```python
from build123d import *

# Parameters (mm, degrees)
SKETCH2_W           = 68.2625
SKETCH2_H           = 52.3875
BOSS_EXTRUDE1_DEPTH = 1.5875
SKETCH3_W           = 38.1
SKETCH3_H           = 3.175
SKETCH3_W_2         = 47.625
SKETCH3_W_3         = 4.7625
SKETCH3_H_2         = 7.9375
SKETCH3_W_4         = 7.9375
SKETCH3_H_3         = 4.7625
BOSS_EXTRUDE2_DEPTH = 7.9375
SKETCH5_W           = 34.925
SKETCH5_H           = 4.7625
BOSS_EXTRUDE3_DEPTH = 7.14375
FILLET1_R           = 1.27
SKETCH6_R           = 2.737420774
BOSS_EXTRUDE4_DEPTH = 6.35
SKETCH7_W           = 15.875
SKETCH7_H           = 12.7
BOSS_EXTRUDE5_DEPTH = 11.1125
SKETCH8_W           = 14.2875
SKETCH8_H           = 9.525
BOSS_EXTRUDE6_DEPTH = 11.1125
SKETCH9_R           = 1.5875
CUT_EXTRUDE1_DEPTH  = 1.5875


with BuildPart() as part:
    # Sketch2 → Boss-Extrude1 (new body)
    with BuildSketch(Plane(origin=(0, 0, 0), x_dir=(1, 0, 0), z_dir=(0, 1, 0))):
        with Locations((34.13125, 26.19375)):
            Rectangle(SKETCH2_W, SKETCH2_H)
    extrude(amount=BOSS_EXTRUDE1_DEPTH)

    # Sketch3 → Boss-Extrude2 (add)
    with BuildSketch(Plane(origin=(0, 1.5875, 0), x_dir=(1, 0, 0), z_dir=(0, 1, 0))):
        with Locations((22.225, 49.2125)):
            Rectangle(SKETCH3_W, SKETCH3_H)
        with Locations((26.9875, 3.743785618)):
            Rectangle(SKETCH3_W_2, SKETCH3_H)
        with Locations((5.56088816, 26.190824392)):
            Rectangle(SKETCH3_W_3, SKETCH3_H_2)
        with Locations((50.20501244, 8.616122464)):
            Rectangle(SKETCH3_W_4, SKETCH3_H_3)
    extrude(amount=BOSS_EXTRUDE2_DEPTH)

    # Sketch5 → Boss-Extrude3 (add)
    with BuildSketch(Plane(origin=(0, 1.5875, 0), x_dir=(1, 0, 0), z_dir=(0, 1, 0))):
        with Locations((22.684927586, 36.331025526)):
            Rectangle(SKETCH5_W, SKETCH5_H)
    extrude(amount=BOSS_EXTRUDE3_DEPTH)

    # Fillet1
    fillet1_edges = [part.edges().sort_by_distance(p)[0] for p in [
        (22.684927586, 8.73125, -33.949775526),
        (22.684927586, 8.73125, -38.712275526),
    ]]
    fillet(fillet1_edges, radius=FILLET1_R)

    # Sketch6 → Boss-Extrude4 (add)
    with BuildSketch(Plane(origin=(0, 1.5875, 0), x_dir=(1, 0, 0), z_dir=(0, 1, 0))):
        with Locations(Location((41.97022767, 42.74270286, 0), (0, 0, 90))):
            Circle(SKETCH6_R)
        with Locations(Location((48.357542809, 42.74270286, 0), (0, 0, 90))):
            Circle(SKETCH6_R)
    extrude(amount=BOSS_EXTRUDE4_DEPTH)

    # Sketch7 → Boss-Extrude5 (add)
    with BuildSketch(Plane(origin=(0, 1.5875, 0), x_dir=(1, 0, 0), z_dir=(0, 1, 0))):
        with Locations((66.675, 15.875)):
            Rectangle(SKETCH7_W, SKETCH7_H)
    extrude(amount=BOSS_EXTRUDE5_DEPTH)

    # Sketch8 → Boss-Extrude6 (add)
    with BuildSketch(Plane(origin=(0, 1.5875, 0), x_dir=(1, 0, 0), z_dir=(0, 1, 0))):
        with Locations((62.70625, 44.45)):
            Rectangle(SKETCH8_W, SKETCH8_H)
    extrude(amount=BOSS_EXTRUDE6_DEPTH)

    # Sketch9 → Cut-Extrude1 (cut)
    with BuildSketch(Plane.XZ):
        with Locations(Location((53.637787609, -2.580775526, 0), (0, 0, 270))):
            Circle(SKETCH9_R)
        with Locations(Location((54.45125, -49.806724474, 0), (0, 0, 21.981959095))):
            Circle(SKETCH9_R)
        with Locations(Location((2.38125, -44.599724474, 0), (0, 0, 270))):
            Circle(SKETCH9_R)
        with Locations(Location((2.38125, -17.167724474, 0), (0, 0, 270))):
            Circle(SKETCH9_R)
    extrude(amount=-CUT_EXTRUDE1_DEPTH, mode=Mode.SUBTRACT)


solid = part.part
```
Verification items for the finished model (mm, model axes). A direction names the side the tool comes from. Coordinates: 2 decimals unless noted, no trailing zeros. Write each loop counter-clockwise with the first axis right and the second up, starting at its lowest first coordinate (ties: lowest second). Pieces come first, ordered by that corner, then holes. Notation, with made-up numbers: (-36, -26.75) - (2, -26.75) arc R21 cw to (2, -2.75) - close; hole circle Ø6 at (70, 71.25). An arc over 180 degrees is marked (long way). Write item = value, one per line.
Q1. Cross-section at D-D (y = 2.5). Give the number of separate pieces and of enclosed holes in the cut face, plus the area to 3 significant figures.
Answer:
separate_pieces = 9
enclosed_holes = 0
area = 899 mm²
Q2. Mould release check, pull along X, two halves, no side actions. Record for faces 4 (the face through (53.67, 0.783, -48.425)), 5 (the face through (22, 9.525, -49)), 6 (the face through (69.85, 7, -44)): released by +X, released by -X, zero draft, split by the parting line, or undercut.
Answer:
face_4 = undercut
face_5 = zero draft
face_6 = released by +X
Q3. Cross-section at B-B (z = -7). Enter the section's corners in (x, y) (1 decimal).
Answer:
outline = (0, 0) - (68.3, 0) - (68.3, 1.6) - (54.2, 1.6) - (54.2, 9.5) - (46.2, 9.5) - (46.2, 1.6) - (0, 1.6) - close
Q4. Access from +Z, -Z, +X, -X, +Y, -Y to the whole of each face (thin tool, end or side, straight path). Record for faces 1 (the face through (50, 9.525, -9)), 2 (the face through (55.562, 7, -44)), 3 (the face through (49.41, 4.72, -45.27)).
Answer:
face_1 = +Z, -Z, -X, +Y
face_2 = +Z, -Z, +Y
face_3 = +Y
Q5. Material ranges on L1, parallel to Z at x = 4, y = 2 (3 decimals); L2, parallel to Z at x = 33, y = 5.75 (3 decimals); L3, parallel to Z at x = 6.5, y = 7.25 (3 decimals), recorded low to high. Write a range as from..to.
Answer:
L1 = -50.8..-47.625, -30.16..-22.222, -5.331..-2.156
L2 = -50.8..-47.625, -38.712..-33.95, -5.331..-2.156
L3 = -50.8..-47.625, -38.712..-33.95, -30.16..-22.222, -5.331..-2.156
Q6. Go/stop test with flat-tipped pins: pin 1 Ø1 at (x, y) = (32, 9.5) entering from +Z; pin 2 Ø5 at (x, z) = (51.5, -9) entering from +Y (3 decimals); pin 3 Ø3.5 at (y, z) = (5, -49.5) entering from +X; pin 4 Ø1 at (x, y) = (47.5, 1.5) entering from +Z. Record where each tip stops, or that it passes through.
Answer:
pin_1 = -2.16
pin_2 = 9.525
pin_3 = 69.85
pin_4 = 0
Q7. Cross-section at C-C (x = 21). Enter the section's corners in (y, z) (1 decimal), plus the area to 3 significant figures.
Answer:
outline = (0, -52.4) - (1.6, -52.4) - (1.6, -50.8) - (9.5, -50.8) - (9.5, -47.6) - (1.6, -47.6) - (1.6, -38.7) - (7.5, -38.7) arc R1.3 ccw to (8.7, -37.4) - (8.7, -35.2) arc R1.3 ccw to (7.5, -33.9) - (1.6, -33.9) - (1.6, -5.3) - (9.5, -5.3) - (9.5, -2.2) - (1.6, -2.2) - (1.6, 0) - (0, 0) - close
area = 167 mm²
